```python
from build123d import *

# Parameters (mm, degrees)
SKETCH1_R           = 2.5
BOSS_EXTRUDE2_DEPTH = 50


with BuildPart() as part:
    # Sketch1 → Boss-Extrude2 (new body)
    with BuildSketch(Plane.XY):
        with BuildLine():
            Line((10, -4.1), (10, -8.5))
            ThreePointArc((10, -8.5), (9.560660172, -9.560660172), (8.5, -10))
            Line((8.5, -10), (4.1, -10))
            Line((4.1, -10), (4.1, -9.5))
            Line((4.1, -9.5), (3.6, -9.5))
            Line((3.6, -9.5), (3.6, -8.2))
            Line((3.6, -8.2), (5.5, -8.2))
            Line((5.5, -8.2), (5.5, -6.560660172))
            Line((5.5, -6.560660172), (3.425126266, -4.485786438))
            ThreePointArc((3.425126266, -4.485786438), (2.776279568, -4.052240935), (2.010912703, -3.9))
            Line((2.010912703, -3.9), (-2.010912703, -3.9))
            ThreePointArc((-2.010912703, -3.9), (-2.776279568, -4.052240935), (-3.425126266, -4.485786438))
            Line((-3.425126266, -4.485786438), (-5.5, -6.560660172))
            Line((-5.5, -6.560660172), (-5.5, -8.2))
            Line((-5.5, -8.2), (-3.6, -8.2))
            Line((-3.6, -8.2), (-3.6, -9.5))
            Line((-3.6, -9.5), (-4.1, -9.5))
            Line((-4.1, -9.5), (-4.1, -10))
            Line((-4.1, -10), (-8.5, -10))
            ThreePointArc((-8.5, -10), (-9.560660172, -9.560660172), (-10, -8.5))
            Line((-10, -8.5), (-10, -4.1))
            Line((-10, -4.1), (-9.5, -4.1))
            Line((-9.5, -4.1), (-9.5, -3.6))
            Line((-9.5, -3.6), (-8.2, -3.6))
            Line((-8.2, -3.6), (-8.2, -5.5))
            Line((-8.2, -5.5), (-6.560660172, -5.5))
            Line((-6.560660172, -5.5), (-4.485786438, -3.425126266))
            ThreePointArc((-4.485786438, -3.425126266), (-4.052240935, -2.776279568), (-3.9, -2.010912703))
            Line((-3.9, -2.010912703), (-3.9, 2.010912703))
            ThreePointArc((-3.9, 2.010912703), (-4.052240935, 2.776279568), (-4.485786438, 3.425126266))
            Line((-4.485786438, 3.425126266), (-6.560660172, 5.5))
            Line((-6.560660172, 5.5), (-8.2, 5.5))
            Line((-8.2, 5.5), (-8.2, 3.6))
            Line((-8.2, 3.6), (-9.5, 3.6))
            Line((-9.5, 3.6), (-9.5, 4.1))
            Line((-9.5, 4.1), (-10, 4.1))
            Line((-10, 4.1), (-10, 8.5))
            ThreePointArc((-10, 8.5), (-9.560660172, 9.560660172), (-8.5, 10))
            Line((-8.5, 10), (-4.1, 10))
            Line((-4.1, 10), (-4.1, 9.5))
            Line((-4.1, 9.5), (-3.6, 9.5))
            Line((-3.6, 9.5), (-3.6, 8.2))
            Line((-3.6, 8.2), (-5.5, 8.2))
            Line((-5.5, 8.2), (-5.5, 6.560660172))
            Line((-5.5, 6.560660172), (-3.425126266, 4.485786438))
            ThreePointArc((-3.425126266, 4.485786438), (-2.776279568, 4.052240935), (-2.010912703, 3.9))
            Line((-2.010912703, 3.9), (2.010912703, 3.9))
            ThreePointArc((2.010912703, 3.9), (2.776279568, 4.052240935), (3.425126266, 4.485786438))
            Line((3.425126266, 4.485786438), (5.5, 6.560660172))
            Line((5.5, 6.560660172), (5.5, 8.2))
            Line((5.5, 8.2), (3.6, 8.2))
            Line((3.6, 8.2), (3.6, 9.5))
            Line((3.6, 9.5), (4.1, 9.5))
            Line((4.1, 9.5), (4.1, 10))
            Line((4.1, 10), (8.5, 10))
            ThreePointArc((8.5, 10), (9.560660172, 9.560660172), (10, 8.5))
            Line((10, 8.5), (10, 4.1))
            Line((10, 4.1), (9.5, 4.1))
            Line((9.5, 4.1), (9.5, 3.6))
            Line((9.5, 3.6), (8.2, 3.6))
            Line((8.2, 3.6), (8.2, 5.5))
            Line((8.2, 5.5), (6.560660172, 5.5))
            Line((6.560660172, 5.5), (4.485786438, 3.425126266))
            ThreePointArc((4.485786438, 3.425126266), (4.052240935, 2.776279568), (3.9, 2.010912703))
            Line((3.9, 2.010912703), (3.9, -2.010912703))
            ThreePointArc((3.9, -2.010912703), (4.052240935, -2.776279568), (4.485786438, -3.425126266))
            Line((4.485786438, -3.425126266), (6.560660172, -5.5))
            Line((6.560660172, -5.5), (8.2, -5.5))
            Line((8.2, -5.5), (8.2, -3.6))
            Line((8.2, -3.6), (9.5, -3.6))
            Line((9.5, -3.6), (9.5, -4.1))
            Line((9.5, -4.1), (10, -4.1))
        make_face()
        Circle(SKETCH1_R, mode=Mode.SUBTRACT)
    extrude(amount=BOSS_EXTRUDE2_DEPTH)


solid = part.part
```
The model under review builds one solid part; all positions refer to its coordinate system, in mm. A direction names the side the tool comes from. Coordinates: 2 decimals unless noted, no trailing zeros. Write each loop counter-clockwise with the first axis right and the second up, starting at its lowest first coordinate (ties: lowest second). Pieces come first, ordered by that corner, then holes.
1) The part is to be moulded in two halves that separate along X. For faces 1 (the face through (10, -6, 25)), 2 (the face through (-6, 10, 25)), 3 (the face through (5.51, -4.45, 24.65)), say which applies: pulls with the +X half, pulls with the -X half, needs draft (parallel to the pull), parting line crosses it, or undercut.
2) Clearance check with flat-ended pins moving along their axes: pin 1 Ø0.7 at (x, z) = (-9, 21.5) entering from -Y; pin 2 Ø3 at (x, z) = (-0.5, 36.5) entering from +Y; pin 3 Ø2 at (y, z) = (0.5, 21) entering from -X. State where each tip first meets the part, or that it passes through.
3) We need section A-A on y = 1.5. State the section outline as (x, z) points.
4) Machinability: for faces 4 (the face through (9.55, 9.57, 24.65)), 5 (the face through (-9, 3.6, 25)), 6 (the face through (2.79, -4.06, 24.65)), 7 (the face through (0, 3.9, 25)), 8 (the face through (5.54, 4.48, 24.65)), which of the approach directions +Z, -Z, +X, -X, +Y, -Y give a long, thin tool a straight path to every point of the face, cutting with its end or side? Answer none if there is none.
5) We need section B-B on x = 0. State the section outline as (y, z) points, then the cut area to 3 significant figures.
6) To check wall thickness, follow probe 1 along X at (y, z) = (7.25, 38.5); probe 2 along Y at (x, z) = (0, 38.5). State the ranges of each line that lie inside material, in increasing order.
Answer list:
1. face 1: pulls with the +X half
1. face 2: needs draft
1. face 3: undercut
2. pin 1: stops at y = -9.99
2. pin 2: stops at y = 3.9
2. pin 3: stops at x = -3.9
3. outline: (-3.9, 0) - (-2, 0) - (-2, 50) - (-3.9, 50) - close; (2, 0) - (3.9, 0) - (3.9, 50) - (2, 50) - close
4. face 4: +Z, -Z, +X, +Y
4. face 5: +Z, -Z, -X
4. face 6: +Z, -Z, -Y
4. face 7: +Z, -Z, +Y
4. face 8: +Z, -Z
5. outline: (-3.9, 0) - (-2.5, 0) - (-2.5, 50) - (-3.9, 50) - close; (2.5, 0) - (3.9, 0) - (3.9, 50) - (2.5, 50) - close
5. area: 140 mm2
6. probe 1: x = -10 to -5.5, 5.5 to 10
6. probe 2: y = -3.9 to -2.5, 2.5 to 3.9
